Geometry: final body of the model. Coordinates: model frame, mm. A direction names the side the tool comes from. Round coordinates to 2 decimals unless told otherwise and drop trailing zeros. Loops run counter-clockwise (first coordinate to the right, second up) from the corner with the lowest first, then second, coordinate; pieces in that order, holes last. Notation, with made-up numbers: M 39,61 L 55,61 A18 cw 55,93 Z; hole C 78,3 d5. An arc over 180 degrees is marked long. Answer as a JSON object with one key per item and string values.
from build123d import *

# Parameters (mm, degrees)
SKETCH1_R               = 3.1
BOSS_EXTRUDE1_DEPTH     = 45
SKETCH2_R               = 1
CUT_EXTRUDE1_DEPTH      = 4.1
CUT_EXTRUDE1_DEPTH_BACK = 4.1
SKETCH3_R               = 5.5
BOSS_EXTRUDE2_DEPTH     = 5


with BuildPart() as part:
    # Sketch1 → Boss-Extrude1 (new body)
    with BuildSketch(Plane.XY):
        Circle(SKETCH1_R)
    extrude(amount=BOSS_EXTRUDE1_DEPTH)

    # Sketch2 → Cut-Extrude1 (cut, two sides)
    with BuildSketch(Plane(origin=(0, 0, 0), x_dir=(0, 0, -1), z_dir=(1, 0, 0))) as cut_extrude1_sk:
        with Locations((-41.5, 0)):
            Circle(SKETCH2_R)
    extrude(amount=CUT_EXTRUDE1_DEPTH, mode=Mode.SUBTRACT)
    extrude(cut_extrude1_sk.sketch, amount=-CUT_EXTRUDE1_DEPTH_BACK, mode=Mode.SUBTRACT)

    # Sketch3 → Boss-Extrude2 (add)
    with BuildSketch(Plane(origin=(0, 0, 0), x_dir=(-1, 0, 0), z_dir=(0, 0, -1))):
        Circle(SKETCH3_R)
    extrude(amount=BOSS_EXTRUDE2_DEPTH)


solid = part.part
1) Section query C-C (z = 41.5). Return the cut outline in (x, y), and give its area (3 significant figures).
Results:
{"outline": "M -2.93,-1 A3.1 ccw 2.93,-1 Z; M -2.93,1 L 2.93,1 A3.1 ccw Z", "area": "18.0 mm2"}
2) Section query D-D (y = 4.5). Return the cut outline in (x, z), and give its area (3 significant figures).
Results:
{"outline": "M -3.16,-5 L 3.16,-5 L 3.16,0 L -3.16,0 Z", "area": "31.6 mm2"}
3) Reachability of faces 1 (the flat face through (0, 0, 45)), 2 (the flat face through (-2.4, -2.4, 0)) from +Z, -Z, +X, -X, +Y, -Y: full face, straight path, thin tool, end or side. Return the list, or none.
Results:
{"face 1": "+Z, +X, -X, +Y, -Y", "face 2": "+Z"}
4) Pin query (flat end, axial travel): P1, Ø4, axis at x = -3, y = 3.5, coming from the +Z side; P2, Ø2, axis at x = 3.5, z = 7.5, coming from the +Y side; P3, Ø1.5, axis at y = 1, z = 1.5, coming from the -X side; P4, Ø1.8, axis at y = 0, z = 41.5, coming from the -X side. Return the tip coordinate at first contact, or that it passes through.
Results:
{"P1": "z = 45", "P2": "y = 1.83", "P3": "x = -3.09", "P4": "through"}
5) Section query B-B (x = -2). Return the cut outline in (y, z).
Results:
{"outline": "M -5.12,-5 L 5.12,-5 L 5.12,0 L 2.37,0 L 2.37,45 L -2.37,45 L -2.37,0 L -5.12,0 Z; hole C 0,41.5 d2"}
6) Section query A-A (y = 0). Return the cut outline in (x, z).
Results:
{"outline": "M -5.5,-5 L 5.5,-5 L 5.5,0 L 3.1,0 L 3.1,40.5 L -3.1,40.5 L -3.1,0 L -5.5,0 Z; M -3.1,42.5 L 3.1,42.5 L 3.1,45 L -3.1,45 Z"}
7) Ray query, line 1 (Z direction, x = 2.1, y = 0); line 2 (Z direction, x = 3.5, y = -0.5); line 3 (Y direction, x = 0.85, z = 41.5). Return the intervals inside material, ascending.
Results:
{"line 1": "-5 to 40.5, 42.5 to 45", "line 2": "-5 to 0", "line 3": "-2.98 to -1, 1 to 2.98"}
